```python
from build123d import *

# Parameters (mm, degrees)
PAD_DEPTH    = 8
SKETCH001_R  = 1.5
PAD001_DEPTH = 6
SKETCH002_R  = 1.5
POCKET_DEPTH = 6


with BuildPart() as part:
    # Sketch → Pad (new body)
    with BuildSketch(Plane.XY):
        Polygon((3, -1.732051), (3, 1.732051), (0, 3.464102), (-3, 1.732051), (-3, -1.732051), (0, -3.464102), align=None)
    extrude(amount=PAD_DEPTH)

    # Sketch001 (on Face7 of Pad) → Pad001 (join)
    with BuildSketch(Plane(origin=(0, 0, 0), x_dir=(1, 0, 0), z_dir=(0, 0, -1))):
        Circle(SKETCH001_R)
    extrude(amount=PAD001_DEPTH)

    # Sketch002 (on Face5 of Pad001) → Pocket (cut)
    with BuildSketch(Plane.XY.offset(8)):
        Circle(SKETCH002_R)
    extrude(amount=-POCKET_DEPTH, mode=Mode.SUBTRACT)


solid = part.part
```
Verification items for the finished model (mm, model axes). A direction names the side the tool comes from. Give positions to 0.01 mm unless a question says otherwise; leave off trailing zeros. Loops run counter-clockwise (first coordinate to the right, second up) from the corner with the lowest first, then second, coordinate; pieces in that order, holes last. Notation, with made-up numbers: M 80,47.25 L 125,47.25 A18 ccw 125,72.25 Z; hole C 24,53 d1. An arc over 180 degrees is marked long. Return JSON: item names as keys, results as strings.
1) Section check C-C, the plane z = 0.5. Enter the section's corners in (x, y).
Findings:
{"outline": "M -3,-1.73 L 0,-3.46 L 3,-1.73 L 3,1.73 L 0,3.46 L -3,1.73 Z"}
2) Section check B-B, the plane y = 0. Enter the section's corners in (x, z).
Findings:
{"outline": "M -3,0 L -1.5,0 L -1.5,-6 L 1.5,-6 L 1.5,0 L 3,0 L 3,8 L 1.5,8 L 1.5,2 L -1.5,2 L -1.5,8 L -3,8 Z"}
3) Material ranges on L1, parallel to Z at x = -0.5, y = 1.75; L2, parallel to Y at x = 0.25, z = 7; L3, parallel to X at y = 0.5, z = 7, recorded low to high. Write a range as [from, to].
Findings:
{"L1": "z = [0, 8]", "L2": "y = [-3.32, -1.48], [1.48, 3.32]", "L3": "x = [-3, -1.41], [1.41, 3]"}
4) Mould release check, pull along X, two halves, no side actions. Record for faces 4 (the flat face through (-1.5, 2.6, 3.9)), 5 (the flat face through (0, 0, -6)), 6 (the flat face through (3, 0, 4)), 7 (the flat face through (0, 0, 2)): released by +X, released by -X, zero draft, split by the parting line, or undercut.
Findings:
{"face 4": "released by -X", "face 5": "zero draft", "face 6": "released by +X", "face 7": "undercut"}
5) Tool access check on faces 1 (the cylindrical face through (-1.5, 0.07, 5.04)), 2 (the cylindrical face through (-1.5, -0.07, -2.96)), 3 (the flat face through (-3, 0, 4)). Record the directions out of +Z, -Z, +X, -X, +Y, -Y that give a thin tool (end or side, any length) a straight path to the whole face; none if there is none.
Findings:
{"face 1": "+Z", "face 2": "-Z", "face 3": "+Z, -Z, -X, +Y, -Y"}
6) Section check A-A, the plane z = 3.75. Enter the section's corners in (x, y), and give its area (3 significant figures).
Findings:
{"outline": "M -3,-1.73 L 0,-3.46 L 3,-1.73 L 3,1.73 L 0,3.46 L -3,1.73 Z; hole C 0,0 d3", "area": "24.1 mm2"}
7) Gauge pin test, flat ends, axial feed: P1, Ø1, axis at x = 0.5, z = -1.5, coming from the +Y side; P2, Ø2, axis at x = 0.5, z = 6.5, coming from the -Y side. Record the tip position at first contact, or that the pin passes through.
Findings:
{"P1": "stops at y = 1.5", "P2": "stops at y = -3.46"}
8) Section check D-D, the plane x = -1. Enter the section's corners in (y, z), and give its area (3 significant figures).
Findings:
{"outline": "M -2.89,0 L -1.12,0 L -1.12,-6 L 1.12,-6 L 1.12,0 L 2.89,0 L 2.89,8 L 1.12,8 L 1.12,2 L -1.12,2 L -1.12,8 L -2.89,8 Z", "area": "46.2 mm2"}
